Autodesk Inventor part; units mm, degrees
ref_plane "Start Plane" through (0, 0, -4.4541) normal (0, 0, 1) x (1, 0, 0)
ref_plane "End Plane" through (0, 0, 219.0092) normal (0, 0, 1) x (1, 0, 0)
ref_plane "Work Plane4" through (-3.2535, -10.1598, -4.8357) normal (0.1259, 0.3932, -0.9108) x (0.8223, -0.555, -0.1259)
ref_plane "Start Plane" through (0, 0, -4.4541) normal (0, 0, 1) x (1, 0, 0)
ref_plane "End Plane" through (0, 0, 219.0092) normal (0, 0, 1) x (1, 0, 0)
sketch "Sketch" plane through (0, 0, 0) normal (0, 0, 1) x (1, 0, 0)
  circle A0 centre (0, 0) radius 6.9342
  circle A1 centre (0, 0) radius 10.668
  dimension "d0" = 21.336
  dimension "d1" = 3.7338
extrude "Body" add sketch "Sketch" along normal up to surface (223.4633 mm away) from surface at -4.4541
sketch "Sketch3" plane through (0, 0, 0) normal (0, 0, 1) x (1, 0, 0)
  line L0 (0, 0) -> (10, 0)
ref_plane "Work Plane3" through (0, 0, 0) normal (0, -1, 0) x (1, 0, 0)
sketch "Sketch4" plane through (0, 0, 0) normal (0, -1, 0) x (1, 0, 0)
  line L0 (-2, -4.4541) -> (12, -4.4541)
  line L1 (-2, 219.0092) -> (12, 219.0092)
  dimension "d7" = 223.4633
ref_plane "Work Plane4" through (-3.2535, -10.1598, -4.8357) normal (0.1259, 0.3932, -0.9108) x (0.8223, -0.555, -0.1259)
split "Split1" plane through (-3.2535, -10.1598, -4.8357) removes the side toward (0.1259, 0.3932, -0.9108)
ref_plane "Work Plane5" through (-7.3135, -7.7665, -10.5353) normal (0.4817, 0.5116, -0.7115) x (0.1956, -0.8542, -0.4817)
split "Split2" plane through (-7.3135, -7.7665, -10.5353) removes the side toward (0.4817, 0.5116, -0.7115)
ref_plane "Work Plane6" through (10.1246, -3.3615, -11.1594) normal (-0.686, 0.2278, -0.691) x (-0.5231, 0.5057, 0.686)
split "Split3" plane through (10.1246, -3.3615, -11.1594) removes the side toward (-0.686, 0.2278, -0.691)
ref_plane "Work Plane7" through (-7.3135, -7.7665, 234.1893) normal (0.6196, 0.658, 0.4281) x (0.7312, -0.2855, -0.6196)
split "Split4" plane through (-7.3135, -7.7665, 234.1893) removes the side toward (0.6196, 0.658, 0.4281)
ref_plane "Work Plane8" through (10.1246, -3.3615, 221.8641) normal (-0.6558, 0.2177, 0.7228) x (0.7504, 0.0829, 0.6558)
split "Split5" plane through (10.1246, -3.3615, 221.8641) removes the side toward (-0.6558, 0.2177, 0.7228)
ref_plane "Work Plane9" through (-4.3247, -9.7521, 225.8384) normal (0.3239, 0.7304, 0.6014) x (0.9345, -0.1477, -0.3239)
split "Split6" plane through (-4.3247, -9.7521, 225.8384) removes the side toward (0.3239, 0.7304, 0.6014)
ref_plane "Work Plane10" through (62.1464, 22.3578, 116.7404) normal (0.6961, -0.706, 0.1304) x (0.3669, 0.506, 0.7806)
sketch "Sketch5" plane through (62.1464, 22.3578, 116.7404) normal (0.6961, -0.706, 0.1304) x (0.3669, 0.506, 0.7806)
  circle A0 centre (4.7916, 74.4945) radius 4
  point P0 (-125.244, -21.9347)
hole "Hole1" at (17.9374, -12.1334, 166.0182) direction (-0.6961, 0.706, -0.1304) diameter 5.4 depth 20 tip angle 118
equation "\"d0\" = G_H"
equation "\"d1\" = G_T"
equation "\"d2\" = G_L"
equation "\"G_H\" = 21.336"
equation "\"G_T\" = 3.7338"
equation "\"G_L\" = 223.46334"
equation "\"G_OFFSET_START\" = 4.45413"
equation "\"G_OFFSET_END\" = 7.34335"
equation "\"d4\" = -G_OFFSET_START"
equation "\"d5\" = G_OFFSET_END + B_L"
equation "\"B_L\" = 211.66586"
properties part number "ANSI - 1/2 x 0.147 - 8.798" material "Steel, Mild"
Input: part model. Units: mm. Frame: model coordinates. Round coordinates to 2 decimals unless told otherwise and drop trailing zeros. Loops run counter-clockwise (first coordinate to the right, second up) from the corner with the lowest first, then second, coordinate; pieces in that order, holes last. Notation, with made-up numbers: (-33.5, 0) -> (-28.5, 0) arc R30 ccw to (-28.5, 30) -> close; hole circle Ø7 at (-1.75, 27.25). An arc over 180 degrees is marked (long way). One line per item, written item: value.
(1) Material intervals for line 1 (Y direction, x = 0, z = 48); line 2 (Z direction, x = 8, y = 1), sorted ascending. Write a range as [from, to].
Geometry check:
line 1: [-10.67, -6.93], [6.93, 10.67]
line 2: [6.14, 162.22], [165.52, 198.55]
(2) Section A-A (z = 183). Return the cut outline in (x, y).
Geometry check:
outline: circle Ø21.34 at (0, 0); hole circle Ø13.87 at (0, 0)
(3) Mould query, pull axis Y, two halves, no side actions, for faces 1 (the face through (9.84, -0.09, 164.39)), 2 (the face through (6.6, 3, 197.5)), 3 (the face through (-1.389, -10.577, 105.713)). Classes: pulls with the +Y half, pulls with the -Y half, needs draft (parallel to the pull), parting line crosses it, or undercut.
Geometry check:
face 1: undercut
face 2: pulls with the +Y half
face 3: parting line crosses it
(4) Pin query (flat end, axial travel): pin 1 (4 mm diameter, centred on y = 5.5, z = 52, fed in from -X); pin 2 (6 mm diameter, centred on y = 7.5, z = 80, fed in from +X); pin 3 (5 mm diameter, centred on x = 3, y = 6, fed in from -Z); pin 4 (8 mm diameter, centred on y = -0.5, z = 103.5, fed in from +X). Return the tip coordinate at first contact, or that it passes through.
Geometry check:
pin 1: x = -10.08
pin 2: x = 9.67
pin 3: z = 5.42
pin 4: x = 10.67
